The drawing under review shows one solid part. Ordinate dimensions are in mm from its lowest x, y, z. A direction names the side the tool comes from. Coordinates: 2 decimals unless noted, no trailing zeros. Loops run counter-clockwise (first coordinate to the right, second up) from the corner with the lowest first, then second, coordinate; pieces in that order, holes last. Notation, with made-up numbers: M 82.5,23.5 L 127.5,23.5 A32 ccw 127.5,52.5 Z; hole C 70.5,15.5 d3. An arc over 180 degrees is marked long. Use one line per item in the form item = value.
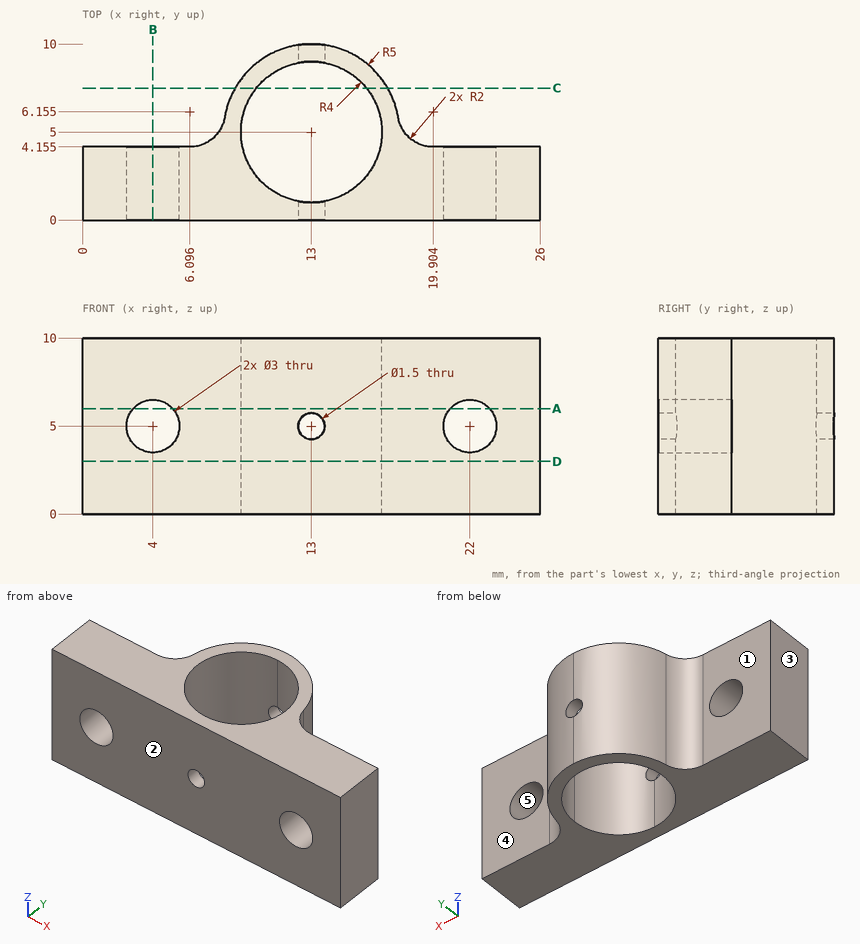
1. Consider section D-D on z = 3. Write out the cut boundary in (x, y) (1 decimal).
Computed values:
outline = M 0,0 L 26,0 L 26,4.2 L 19.9,4.2 A2 cw 17.9,5.8 A5 ccw 8.1,5.8 A2 cw 6.1,4.2 L 0,4.2 Z; hole C 13,5 d8
2. Consider section C-C on y = 7.5. Write out the cut boundary in (x, z).
Computed values:
outline = M 8.67,0 L 9.88,0 L 9.88,10 L 8.67,10 Z; M 16.12,0 L 17.33,0 L 17.33,10 L 16.12,10 Z
3. Consider section B-B on x = 4. Write out the cut boundary in (y, z) (3 decimals).
Computed values:
outline = M 0,0 L 4.155,0 L 4.155,3.5 L 0,3.5 Z; M 0,6.5 L 4.155,6.5 L 4.155,10 L 0,10 Z
4. For pin 1 Ø0.9 at (x, z) = (13, 5) entering from -Y; pin 2 Ø4 at (y, z) = (7.5, 4) entering from +X; pin 3 Ø1.8 at (x, z) = (3.5, 6) entering from +Y (3 decimals); pin 4 Ø1 at (y, z) = (8, 8) entering from -X, all flat-tipped, find the tip position at first contact; note any pin that passes through.
Computed values:
pin_1 = through
pin_2 = 18.01
pin_3 = 4.155
pin_4 = 8.67
5. Consider section A-A on z = 6. Write out the cut boundary in (x, y) (1 decimal).
Computed values:
outline = M 0,0 L 2.9,0 L 2.9,4.2 L 0,4.2 Z; M 5.1,0 L 20.9,0 L 20.9,4.2 L 19.9,4.2 A2 cw 17.9,5.8 A5 ccw 8.1,5.8 A2 cw 6.1,4.2 L 5.1,4.2 Z; M 23.1,0 L 26,0 L 26,4.2 L 23.1,4.2 Z; hole C 13,5 d8
6. Draft analysis for pull direction X (two halves, no side actions). For the marked faces 3, 4 and 5, state which applies: +X half, -X half, draft (parallel to the pull), parting line (faces both ways), or undercut.
Computed values:
face_3 = -X half
face_4 = draft
face_5 = undercut
7. Tool access review of the marked faces 1 and 2: name each direction out of +Z, -Z, +X, -X, +Y, -Y from which nothing blocks a thin tool from reaching the whole face with its end or side.
Computed values:
face_1 = +Z, -Z, -X, +Y
face_2 = +Z, -Z, +X, -X, -Y
8. Wall thickness on line 1 along X through (y, z) = (0.9, 5); line 2 along X through (y, z) = (0.5, 4.5); line 3 along Z through (x, y) = (13, 0.4): over which ranges is each line inside the solid? List them lowest first. Write a range as from..to.
Computed values:
line_1 = 0..2.5, 5.5..12.25, 13.75..20.5, 23.5..26
line_2 = 0..2.59, 5.41..12.44, 13.56..20.59, 23.41..26
line_3 = 0..4.25, 5.75..10
